Design review of the part built by this model. Coordinates are the model's own, in mm. A direction names the side the tool comes from. Coordinates: 2 decimals unless noted, no trailing zeros. Write each loop counter-clockwise with the first axis right and the second up, starting at its lowest first coordinate (ties: lowest second). Pieces come first, ordered by that corner, then holes.
Q1. Take a section at C-C, the plane y = -168.5. Write out the cut boundary in (x, z).
Q2. For L1, parallel to X at y = -161, z = -0.5; L2, parallel to Z at x = -35, y = -148; L3, parallel to Z at x = -169, y = -137, list the stretches that pass through material, from the lowest coordinate up.
Q3. Take a section at B-B, the plane y = -20. Write out the cut boundary in (x, z), plus the area to 3 significant figures.
Q4. The part is to be moulded in two halves that separate along Z. For faces 1 (the flat face through (-250, -47, 45)), 2 (the cylindrical face through (-220.49, -134.3, -55.72)), 3 (the cylindrical face through (-196.474, -88.865, 1.165)), say which applies: released by +Z, released by -Z, zero draft, split by the parting line, or undercut.
Q5. Take a section at D-D, the plane z = 0. Write out the cut boundary in (x, y).
Q6. For pin 1 Ø2.5 at (x, y) = (-42, -133.5) entering from +Z; pin 2 Ø5 at (x, y) = (-132, -15) entering from -Z; pin 3 Ø4 at (y, z) = (-56.5, 59) entering from -X, all flat-tipped, find the tip position at first contact; note any pin that passes through.
Q7. For faces 4 (the cylindrical face through (-247.15, -46.98, 71.99)), 5 (the cylindrical face through (-57.111, -187.465, 20.275)), 6 (the cylindrical face through (20.49, -134.3, 55.72)), list the 3-axis set-ups (+Z, -Z, +X, -X, +Y, -Y) from which the entire face can be reached by the end or side of a thin tool; tool diameter is ignored.
Q8. Take a section at A-A, the plane x = 165. Write out the cut boundary in (y, z).
from build123d import *

# Parameters (mm, degrees)
SKETCH1_W           = 520
SKETCH1_H           = 170
BOSS_EXTRUDE1_DEPTH = 10
BOSS_EXTRUDE2_DEPTH = 75
BOSS_EXTRUDE3_DEPTH = 100
SKETCH4_W           = 7.501461654
SKETCH4_H           = 40
BOSS_EXTRUDE4_DEPTH = 25
SKETCH5_R           = 3.75
CUT_EXTRUDE1_DEPTH  = 93
SKETCH6_W           = 50
SKETCH6_H           = 75
BOSS_EXTRUDE5_DEPTH = 5
SKETCH7_R           = 30
CUT_EXTRUDE2_DEPTH  = 68
SKETCH8_W           = 75
SKETCH8_H           = 75
BOSS_EXTRUDE6_DEPTH = 15
SKETCH9_R           = 30
SKETCH9_R_2         = 26.5
BOSS_EXTRUDE7_DEPTH = 5
SKETCH11_R          = 26.5
CUT_EXTRUDE3_DEPTH  = 75
SKETCH12_R          = 26.5
CUT_EXTRUDE4_DEPTH  = 196
SKETCH14_R          = 7.5
BOSS_EXTRUDE8_DEPTH = 10
CHAMFER1_SIZE       = 3
SKETCH15_R          = 2.5
BOSS_EXTRUDE9_DEPTH = 5


with BuildPart() as part:
    # Sketch1 → Boss-Extrude1 (new body, symmetric)
    with BuildSketch(Plane(origin=(0, 0, 0), x_dir=(1, 0, 0), z_dir=(0, 1, 0))):
        Rectangle(SKETCH1_W, SKETCH1_H)
    extrude(amount=BOSS_EXTRUDE1_DEPTH, both=True)

    # Sketch2 → Boss-Extrude2 (add)
    with BuildSketch(Plane.XZ.offset(10)):
        with BuildLine():
            Line((-240, 75), (40, 75))
            ThreePointArc((40, 75), (47.071067812, 72.071067812), (50, 65))
            Line((50, 65), (50, -65))
            ThreePointArc((50, -65), (47.071067812, -72.071067812), (40, -75))
            Line((40, -75), (-240, -75))
            ThreePointArc((-240, -75), (-247.071067812, -72.071067812), (-250, -65))
            Line((-250, -65), (-250, 65))
            ThreePointArc((-250, 65), (-247.071067812, 72.071067812), (-240, 75))
        make_face()
    extrude(amount=BOSS_EXTRUDE2_DEPTH)

    # Sketch3 → Boss-Extrude3 (add)
    with BuildSketch(Plane.XZ.offset(85)):
        with BuildLine():
            Line((-210, 60), (10, 60))
            ThreePointArc((10, 60), (20.606601718, 55.606601718), (25, 45))
            Line((25, 45), (25, -45))
            ThreePointArc((25, -45), (20.606601718, -55.606601718), (10, -60))
            Line((10, -60), (-210, -60))
            ThreePointArc((-210, -60), (-220.606601718, -55.606601718), (-225, -45))
            Line((-225, -45), (-225, 45))
            ThreePointArc((-225, 45), (-220.606601718, 55.606601718), (-210, 60))
        make_face()
    extrude(amount=BOSS_EXTRUDE3_DEPTH)

    # Sketch4 → Boss-Extrude4 (add)
    with BuildSketch(Plane.ZY.offset(225)):
        with Locations((13.750730827, -135)):
            Rectangle(SKETCH4_W, SKETCH4_H)
        with Locations((-13.750730827, -135)):
            Rectangle(SKETCH4_W, SKETCH4_H)
    extrude(amount=BOSS_EXTRUDE4_DEPTH)

    # Sketch5 → Cut-Extrude1 (cut)
    with BuildSketch(Plane(origin=(0, 0, -17.501461654), x_dir=(-1, 0, 0), z_dir=(0, 0, -1))):
        with Locations((235, -135)):
            Circle(SKETCH5_R)
    extrude(amount=-CUT_EXTRUDE1_DEPTH, mode=Mode.SUBTRACT)

    # Sketch6 → Boss-Extrude5 (add)
    with BuildSketch(Plane.ZY.offset(250)):
        with Locations((0, -47.5)):
            Rectangle(SKETCH6_W, SKETCH6_H)
    extrude(amount=BOSS_EXTRUDE5_DEPTH)

    # Sketch7 → Cut-Extrude2 (cut)
    with BuildSketch(Plane.XZ.offset(10)):
        with Locations((165, 0)):
            Circle(SKETCH7_R)
    extrude(amount=-CUT_EXTRUDE2_DEPTH, mode=Mode.SUBTRACT)

    # Sketch8 → Boss-Extrude6 (add)
    with BuildSketch(Plane(origin=(50, 0, 0), x_dir=(0, 0, -1), z_dir=(1, 0, 0))):
        with Locations((0, -47.5)):
            Rectangle(SKETCH8_W, SKETCH8_H)
    extrude(amount=BOSS_EXTRUDE6_DEPTH)

    # Sketch9 → Boss-Extrude7 (add)
    with BuildSketch(Plane.XZ.offset(185)):
        with Locations((-35, 0)):
            Circle(SKETCH9_R)
        with Locations((-35, 0)):
            Circle(SKETCH9_R_2, mode=Mode.SUBTRACT)
    extrude(amount=BOSS_EXTRUDE7_DEPTH)

    # Sketch11 → Cut-Extrude3 (cut)
    with BuildSketch(Plane.XZ.offset(185)):
        with Locations((-35, 0)):
            Circle(SKETCH11_R)
    extrude(amount=-CUT_EXTRUDE3_DEPTH, mode=Mode.SUBTRACT)

    # Sketch12 → Cut-Extrude4 (cut, through all)
    with BuildSketch(Plane.XZ.offset(185)):
        with Locations((-170, 0)):
            Circle(SKETCH12_R)
    extrude(amount=-CUT_EXTRUDE4_DEPTH, mode=Mode.SUBTRACT)

    # Sketch14 → Boss-Extrude8 (add)
    with BuildSketch(Plane.XY.offset(60)):
        with Locations((-40, -135)):
            Circle(SKETCH14_R)
    extrude(amount=BOSS_EXTRUDE8_DEPTH)

    # Chamfer1
    chamfer1_edges = [part.edges().sort_by_distance(p)[0] for p in [
        (-47.5, -135, 70),
    ]]
    chamfer(chamfer1_edges, length=CHAMFER1_SIZE)

    # Sketch15 → Boss-Extrude9 (add)
    with BuildSketch(Plane.XY.offset(60)):
        with Locations((-170, -135)):
            Circle(SKETCH15_R)
    extrude(amount=BOSS_EXTRUDE9_DEPTH)


solid = part.part
Responses:
1. outline: (-225, -45) arc R15 ccw to (-210, -60) - (10, -60) arc R15 ccw to (25, -45) - (25, 45) arc R15 ccw to (10, 60) - (-210, 60) arc R15 ccw to (-225, 45) - close; hole circle Ø53 at (-170, 0); hole circle Ø53 at (-35, 0)
2. L1: x = -225 to -196.5, -143.5 to -61.5, -8.5 to 25
2. L2: z = -60 to -26.5, 26.5 to 60
2. L3: z = -60 to -26.48, 26.48 to 65
3. outline: (-255, -25) - (-250, -25) - (-250, -65) arc R10 ccw to (-240, -75) - (40, -75) arc R10 ccw to (50, -65) - (50, -37.5) - (65, -37.5) - (65, 37.5) - (50, 37.5) - (50, 65) arc R10 ccw to (40, 75) - (-240, 75) arc R10 ccw to (-250, 65) - (-250, 25) - (-255, 25) - close; hole circle Ø53 at (-170, 0)
3. area: 44,100 mm2
4. face 1: zero draft
4. face 2: released by -Z
4. face 3: undercut
5. outline: (-260, -10) - (-255, -10) - (-255, -85) - (-225, -85) - (-225, -185) - (-196.5, -185) - (-196.5, 10) - (-260, 10) - close; (-143.5, -185) - (-65, -185) - (-65, -190) - (-61.5, -190) - (-61.5, -110) - (-8.5, -110) - (-8.5, -190) - (-5, -190) - (-5, -185) - (25, -185) - (25, -85) - (65, -85) - (65, -10) - (135, -10) - (135, 10) - (-143.5, 10) - close; (195, -10) - (260, -10) - (260, 10) - (195, 10) - close
6. pin 1: stops at z = 70
6. pin 2: stops at z = -75
6. pin 3: stops at x = -250
7. face 4: +Z, -X, -Y
7. face 5: -Y
7. face 6: +Z, +X, -Y
8. outline: (-10, -85) - (10, -85) - (10, -30) - (-10, -30) - close; (-10, 30) - (10, 30) - (10, 85) - (-10, 85) - close
